from build123d import *

# Parameters (mm, degrees)
F1_DEPTH = 25
F2_R     = 2


with BuildPart() as f1:
    # F0 (on Top) → F1 (new body)
    with BuildSketch(Plane.XY):
        Polygon((6.565958, 37.105379), (-23.434042, 37.105379), (-63.434042, 7.105379), (-23.434042, 7.105379), (6.565958, 7.105379), align=None)
    extrude(amount=F1_DEPTH)

    # F2
    f2_edges = [f1.edges().sort_by_distance(p)[0] for p in [
        (-28.434042, 7.105379, 25),
        (6.565958, 22.105379, 25),
        (-8.434042, 37.105379, 25),
        (-43.434042, 22.105379, 25),
        (6.565958, 7.105379, 12.5),
        (-28.434042, 7.105379, 0),
        (-63.434042, 7.105379, 12.5),
        (-23.434042, 37.105379, 12.5),
        (-43.434042, 22.105379, 0),
        (6.565958, 37.105379, 12.5),
        (-8.434042, 37.105379, 0),
        (6.565958, 22.105379, 0),
    ]]
    fillet(f2_edges, radius=F2_R)


solid = f1.part
Build history of the part. All positions in model axes, mm. Round coordinates to 2 decimals unless told otherwise and drop trailing zeros. Order: outer loops, then holes, each group sorted by start corner. A loop starts at its lowest first (then second) coordinate and runs counter-clockwise, first axis right, second up. Notation, with made-up numbers: M -29.75,-2 L -17.75,-2 A23 ccw -17.75,17 Z; hole C 77.5,79.5 d8. An arc over 180 degrees is marked long. Use CSV: the item, a comma, the result in double quotes. Start each with the question number.
(1) Cut at A-A on z = 7.75. List the corners of the cut face in (x, y), then the cut area to 3 significant figures.
(2) Flat gauge pins, fed straight in: P1, Ø1, axis at x = -48.5, z = 8, coming from the +Y side; P2, Ø4, axis at y = 32, z = 10, coming from the -X side; P3, Ø2, axis at x = -30, y = 32, coming from the +Z side. Where does each tip first touch, or does it go through?
(3) Drill centre lines: probe 1 along Z at (x, y) = (-7, 36); probe 2 along X at (y, z) = (12, 6); probe 3 along X at (y, z) = (9.5, 13.75). Where is each one in solid material? Low to high.
Findings:
1,outline,"M -58.63,10.71 A2 ccw -57.43,7.11 L 4.57,7.11 A2 ccw 6.57,9.11 L 6.57,35.11 A2 ccw 4.57,37.11 L -22.77,37.11 A2 ccw -23.97,36.71 Z"
1,area,"1,490 mm^2"
2,P1,"stops at y = 18.68"
2,P2,"stops at x = -32.91"
2,P3,"stops at z = 24.81"
3,probe 1,"z = 0.21 to 24.79"
3,probe 2,"x = -56.91 to 6.57"
3,probe 3,"x = -59.39 to 6.57"
